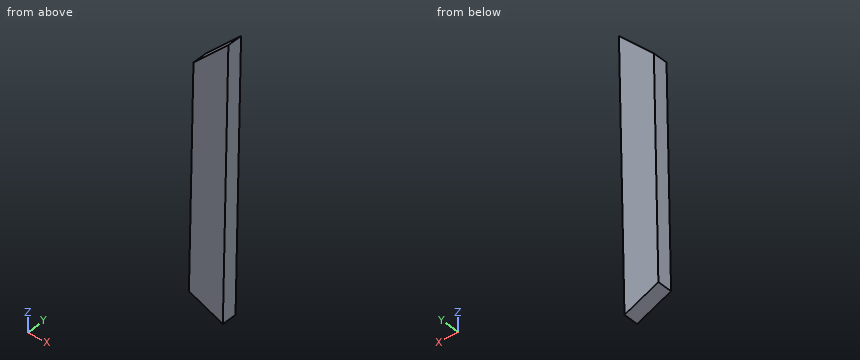
Autodesk Inventor part; units mm, degrees
ref_plane "YZ Plane" through (0, 0, 0) normal (1, 0, 0) x (0, 1, 0)
ref_plane "XZ Plane" through (0, 0, 0) normal (0, 1, 0) x (-1, 0, 0)
ref_plane "XY Plane" through (0, 0, 0) normal (0, 0, 1) x (1, 0, 0)
sketch "Sketch1" plane through (0, 0, 0) normal (0, 1, 0) x (-1, 0, 0)
  line L0 (0, 0) -> (0, -1219.2)
  line L1 (0, 0) -> (88.9, 0)
  line L2 (88.9, 0) -> (88.9, -1219.2)
  line L3 (88.9, -1219.2) -> (0, -1219.2)
  line L4 (0, 0) -> (0, 1219.2) construction
  line L5 (0, 1219.2) -> (1219.2, 1219.2) construction
  line L6 (0, 1219.2) -> (0, 3657.6) construction
  line L7 (0, 3657.6) -> (0, 4876.8) construction
  line L8 (0, 4876.8) -> (0, 6096) construction
  line L9 (0, -1219.2) -> (2438.4, -1219.2) construction
  line L10 (0, 6096) -> (2438.4, 6096) construction
  line L11 (2438.4, 6096) -> (2438.4, -1219.2) construction
  line L12 (0, 3657.6) -> (0, 3352.8) construction
  line L13 (0, 3352.8) -> (2438.4, 3352.8) construction
  line L14 (2438.4, 3352.8) -> (1219.2, 3352.8)
  line L15 (1219.2, 3352.8) -> (1219.2, 3263.9)
  line L16 (1219.2, 3263.9) -> (2438.4, 3263.9)
  line L17 (2438.4, 3263.9) -> (2438.4, 3352.8)
  line L18 (0, 6096) -> (862.1046, 6958.1046)
  line L19 (862.1046, 6958.1046) -> (924.9664, 6895.2428)
  line L20 (924.9664, 6895.2428) -> (62.8618, 6033.1382)
  line L21 (62.8618, 6033.1382) -> (0, 6096)
  line L22 (0, 4876.8) -> (1219.2, 4876.8) construction
  line L23 (1219.2, 4876.8) -> (2081.3046, 5738.9046)
  line L24 (1219.2, 1219.2) -> (2081.3046, 357.0954)
  line L25 (2081.3046, 357.0954) -> (2018.4428, 294.2336)
  line L26 (2018.4428, 294.2336) -> (1156.3382, 1156.3382)
  line L27 (1156.3382, 1156.3382) -> (1219.2, 1219.2)
  line L28 (2018.4428, 294.2336) -> (88.9, -1219.2)
  line L29 (2081.3046, 357.0954) -> (2144.1664, 419.9572)
  line L30 (2144.1664, 419.9572) -> (1282.0618, 1282.0618)
  line L31 (1282.0618, 1282.0618) -> (1219.2, 1219.2)
  line L32 (2438.4, 3352.8) -> (2438.4, 3441.7)
  line L33 (2438.4, 3441.7) -> (1219.2, 3441.7)
  line L34 (1219.2, 3441.7) -> (1219.2, 3352.8)
  line L35 (1156.3382, 4939.6618) -> (1282.0618, 4813.9382)
  line L36 (2018.4428, 5801.7664) -> (2144.1664, 5676.0428)
  line L37 (1282.0618, 4813.9382) -> (2144.1664, 5676.0428)
  line L38 (2018.4428, 5801.7664) -> (1156.3382, 4939.6618)
  line L39 (2018.4428, 5801.7664) -> (924.9664, 6895.2428)
  line L40 (62.8618, 6033.1382) -> (1156.3382, 4939.6618)
  line L41 (1233.6206, 4168.8855) -> (1267.6412, 4086.7527)
  line L42 (1263.7078, 2313.9849) -> (1230.0006, 2231.7229)
  arc A0 (862.1046, 6958.1046) -> (0, 6096) centre (431.0523, 6527.0523) ccw
  line L43 (1246.8542, 2272.8539) -> (2375.0183, 1810.583)
  line L44 (2391.8719, 1851.7139) -> (2358.1646, 1769.452)
  line L45 (2391.8719, 1851.7139) -> (1263.7078, 2313.9849)
  line L46 (1230.0006, 2231.7229) -> (2358.1646, 1769.452)
  line L47 (1230.0006, 2231.7229) -> (1219.2, 3263.9)
  line L48 (2144.1664, 419.9572) -> (2391.8719, 1851.7139)
  line L49 (2391.8719, 1851.7139) -> (2438.4, 3263.9)
  line L50 (1219.2, 3441.7) -> (1233.6206, 4168.8855)
  line L51 (1250.6309, 4127.8191) -> (2377.0248, 4594.3867)
  line L52 (2360.0145, 4635.4532) -> (2394.0351, 4553.3203)
  line L53 (2394.0351, 4553.3203) -> (1267.6412, 4086.7527)
  line L54 (2360.0145, 4635.4532) -> (1233.6206, 4168.8855)
  line L55 (2394.0351, 4553.3203) -> (2144.1664, 5676.0428)
  line L56 (2438.4, 3441.7) -> (2394.0351, 4553.3203)
  line L57 (2144.1664, 5676.0428) -> (2057.3895, 5656.7301)
  line L58 (2394.0351, 4553.3203) -> (2305.2058, 4549.7751)
  line L59 (2394.0351, 4553.3203) -> (2307.2582, 4534.0076)
  line L60 (2307.2582, 4534.0076) -> (2057.3895, 5656.7301)
  line L61 (2438.4, 3441.7) -> (2349.5707, 3438.1548)
  line L62 (2349.5707, 3438.1548) -> (2305.2058, 4549.7751)
  line L63 (1219.2, 3441.7) -> (1308.0825, 3439.9374)
  line L64 (1233.6206, 4168.8855) -> (1322.5031, 4167.1229)
  line L65 (1322.5031, 4167.1229) -> (1308.0825, 3439.9374)
  line L66 (2018.4428, 5801.7664) -> (1955.581, 5738.9046)
  line L67 (1955.581, 5738.9046) -> (862.1046, 6832.381)
  line L68 (924.9664, 6895.2428) -> (862.1046, 6832.381)
  line L69 (62.8618, 6033.1382) -> (125.7236, 6096)
  line L70 (62.8618, 6033.1382) -> (125.7236, 6096)
  line L71 (125.7236, 6096) -> (1219.2, 5002.5236)
  line L72 (1156.3382, 1156.3382) -> (0, 0)
  line L73 (0, 0) -> (62.8618, -62.8618)
  line L74 (1156.3382, 1156.3382) -> (1219.2, 1093.4764)
  line L75 (1219.2, 1093.4764) -> (62.8618, -62.8618)
  line L76 (2018.4428, 294.2336) -> (1963.5776, 364.1837)
  line L77 (88.9, -1219.2) -> (34.0348, -1149.2499)
  line L78 (34.0348, -1149.2499) -> (1963.5776, 364.1837)
  line L79 (2144.1664, 419.9572) -> (2056.5677, 435.1125)
  line L80 (2391.8719, 1851.7139) -> (2304.2732, 1866.8692)
  line L81 (2391.8719, 1851.7139) -> (2303.0201, 1854.6414)
  line L82 (2304.2732, 1866.8692) -> (2056.5677, 435.1125)
  line L83 (1230.0006, 2231.7229) -> (1318.8957, 2232.6531)
  line L84 (1219.2, 3263.9) -> (1308.0951, 3264.8302)
  line L85 (1308.0951, 3264.8302) -> (1318.8957, 2232.6531)
  line L86 (2438.4, 3263.9) -> (2349.5482, 3266.8275)
  line L87 (2349.5482, 3266.8275) -> (2303.0201, 1854.6414)
  line L88 (88.9, 0) -> (125.7236, 0)
  line L89 (1233.6206, 4168.8855) -> (1219.2, 4876.8)
  line L90 (1233.6206, 4168.8855) -> (1322.5022, 4170.6961)
  line L91 (1219.2, 4876.8) -> (1308.0816, 4878.6106)
  line L92 (1308.0816, 4878.6106) -> (1322.5022, 4170.6961)
  line L93 (1282.0618, 4813.9382) -> (1309.9674, 4786.0326)
  line L94 (1267.6412, 4086.7527) -> (1318.4756, 3964.0275)
  line L95 (2360.0145, 4635.4532) -> (2374.4273, 4641.4231)
  line L96 (1230.0006, 2231.7229) -> (1219.2, 1219.2)
  line L97 (1230.0006, 2231.7229) -> (1318.8955, 2230.7747)
  line L98 (1219.2, 1219.2) -> (1308.0949, 1218.2518)
  line L99 (1308.0949, 1218.2518) -> (1318.8955, 2230.7747)
  line L100 (1282.0618, 1282.0618) -> (1309.0636, 1309.0636)
  line L101 (1263.7078, 2313.9849) -> (1316.7428, 2438.4)
  line L102 (2358.1646, 1769.452) -> (2376.5379, 1763.082)
  point P0 (1770.957, 2057.4547)
  point P1 (1955.1236, 357.5528)
  point P2 (88.9, -1106.2164)
  point P3 (2292.1025, 1796.5213)
  point P4 (2067.2525, 496.8711)
  point P5 (1318.5187, 2195.4522)
  point P6 (1308.1049, 3263.9)
  point P7 (2349.4518, 3263.9)
  point P8 (2304.1085, 1887.6754)
  point P9 (2306.5112, 4517.0667)
  point P10 (2349.4292, 3441.7)
  point P11 (1308.1175, 3441.7)
  point P12 (2069.6708, 5601.5472)
  point P13 (2291.0394, 4606.8827)
  point P14 (1321.7951, 4205.4086)
  dimension "d0" = 1219.2
  dimension "d2" = 1219.2
  dimension "d3" = 1219.2
  dimension "d16" = 2438.4
  dimension "d17" = 1219.2
  dimension "d18" = 1219.2
  dimension "d20" = 2438.4
  dimension "d21" = 304.8
  dimension "d22" = 1219.2
  dimension "d23" = 88.9
  dimension "d24" = 1219.2
  dimension "d25" = 45
  dimension "d26" = 88.9
  dimension "d27" = 1219.2
  dimension "d28" = 1219.2
  dimension "d29" = 1219.2
  dimension "d31" = 1219.2
  dimension "d32" = 88.9
  dimension "d33" = 88.9
  dimension "d34" = 88.9
  dimension "d35" = 177.8
  dimension "d36" = 177.8
  dimension "d38" = 88.9
  dimension "d39" = 88.9
  dimension "d43" = 1219.2
  dimension "d44" = 88.9
  dimension "d45" = 1219.2
  dimension "d46" = 88.9
  dimension "d47" = 88.9
  dimension "d48" = 88.9
  dimension "d49" = 88.9
  dimension "d50" = 88.9
  dimension "d51" = 88.9
  dimension "d54" = 88.9
  dimension "d55" = 88.9
  dimension "d57" = 88.9
  dimension "d58" = 88.9
  dimension "d59" = 88.9
  dimension "d60" = 88.9
  dimension "d61" = 88.9
  dimension "d64" = 88.9
  dimension "d65" = 88.9
  dimension "d66" = 88.9
  dimension "d69" = 88.9
  dimension "d70" = 88.9
  dimension "d71" = 88.9
  dimension "d72" = 88.9
extrude "Extrusion1" add sketch "Sketch1" along normal blind 38.1 contours L89 L35 L93 L92 L54
properties part number "S_2x4x27.876"
The model under review builds one solid part; all positions refer to its coordinate system, in mm. Round coordinates to 2 decimals unless told otherwise and drop trailing zeros. Order: outer loops, then holes, each group sorted by start corner. A loop starts at its lowest first (then second) coordinate and runs counter-clockwise, first axis right, second up.
Item 1: Add section A-A, the plane y = 15. State the section outline as (x, z) points, and give its area (3 significant figures).
Working result:
outline: (-1321.8, 4205.41) - (-1233.62, 4168.89) - (-1219.2, 4876.8) - (-1309.97, 4786.03) - close
area: 57,300 mm2
Item 2: To check wall thickness, follow probe 1 along X at (y, z) = (6, 4554.5); probe 2 along X at (y, z) = (16, 4445.5); probe 3 along Z at (x, y) = (-1270.5, 21). State the ranges of each line that lie inside material, in increasing order.
Working result:
probe 1: x = -1314.68 to -1225.77
probe 2: x = -1316.9 to -1227.99
probe 3: z = 4184.16 to 4825.5
Item 3: For pin 1 (1 mm diameter, centred on y = 33, z = 4484, fed in from -X); pin 2 (1 mm diameter, centred on x = -1268, y = 17, fed in from +Z); pin 3 (8 mm diameter, centred on y = 26, z = 4475, fed in from +X), all flat-tipped, find the tip position at first contact; note any pin that passes through.
Working result:
pin 1: stops at x = -1316.13
pin 2: stops at z = 4828.5
pin 3: stops at x = -1227.3
Item 4: Add section B-B, the plane x = -1291. State the section outline as (y, z) points, and give its area (3 significant figures).
Working result:
outline: (0, 4192.65) - (38.1, 4192.65) - (38.1, 4805) - (0, 4805) - close
area: 23,300 mm2
